Here's the drawing with two shaded views (mm, measured from the low corner). I have some questions. A direction names the side the tool comes from. Round coordinates to 2 decimals unless told otherwise and drop trailing zeros. Loops run counter-clockwise (first coordinate to the right, second up) from the corner with the lowest first, then second, coordinate; pieces in that order, holes last.
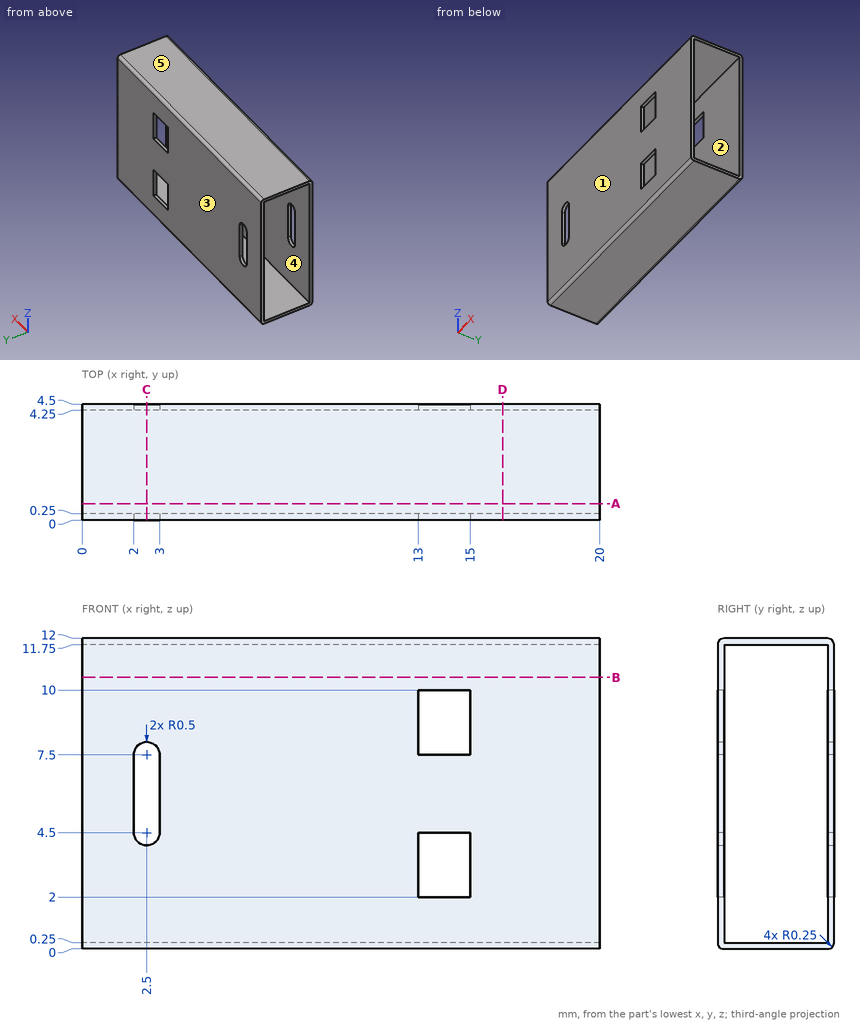
(1) For the marked faces 1 and 2, which set-ups out of +Z, -Z, +X, -X, +Y, -Y let a thin tool reach every point of the face, with its end or its side?
Worked answers:
face 1: +Z, -Z, +X, -X, -Y
face 2: +X, -X
(2) If I drill on line 1 (Z direction, x = 5.5, y = 4.2); line 2 (Y direction, x = 6, z = 10.75), over which ranges is the centre line in solid material (lowest first)?
Worked answers:
line 1: z = 0 to 0.25, 11.75 to 12
line 2: y = 0 to 0.25, 4.25 to 4.5
(3) If we mould it in two halves opening along Y, with no side actions, what happens to the marked faces 3, 4 and 5? For each: released by +Y, released by -Y, zero draft, split by the parting line, or undercut.
Worked answers:
face 3: released by +Y
face 4: undercut
face 5: zero draft
(4) Will this pin go through, and if not, where does the flat tip stop? P1, Ø1, axis at y = 2.5, z = 4.5, coming from the +X side.
Worked answers:
P1: passes through
(5) If we section it at B-B, the plane z = 10.5: List the corners of the cut face in (x, y) for me.
Worked answers:
outline: (0, 0) - (20, 0) - (20, 0.25) - (0, 0.25) - close; (0, 4.25) - (20, 4.25) - (20, 4.5) - (0, 4.5) - close
(6) If we section it at A-A, the plane y = 0.65: List the corners of the cut face in (x, z) for me.
Worked answers:
outline: (0, 0) - (20, 0) - (20, 0.25) - (0, 0.25) - close; (0, 11.75) - (20, 11.75) - (20, 12) - (0, 12) - close
(7) If we section it at D-D, the plane x = 16.25: List the corners of the cut face in (y, z) for me, then the cut area to 3 significant figures.
Worked answers:
outline: (0, 0.25) arc R0.25 ccw to (0.25, 0) - (4.25, 0) arc R0.25 ccw to (4.5, 0.25) - (4.5, 11.75) arc R0.25 ccw to (4.25, 12) - (0.25, 12) arc R0.25 ccw to (0, 11.75) - close; hole (0.25, 0.25) - (4.25, 0.25) - (4.25, 11.75) - (0.25, 11.75) - close
area: 7.95 mm2
(8) If we section it at C-C, the plane x = 2.5: List the corners of the cut face in (y, z) for me.
Worked answers:
outline: (0, 0.25) arc R0.25 ccw to (0.25, 0) - (4.25, 0) arc R0.25 ccw to (4.5, 0.25) - (4.5, 4) - (4.25, 4) - (4.25, 0.25) - (0.25, 0.25) - (0.25, 4) - (0, 4) - close; (0, 8) - (0.25, 8) - (0.25, 11.75) - (4.25, 11.75) - (4.25, 8) - (4.5, 8) - (4.5, 11.75) arc R0.25 ccw to (4.25, 12) - (0.25, 12) arc R0.25 ccw to (0, 11.75) - close
